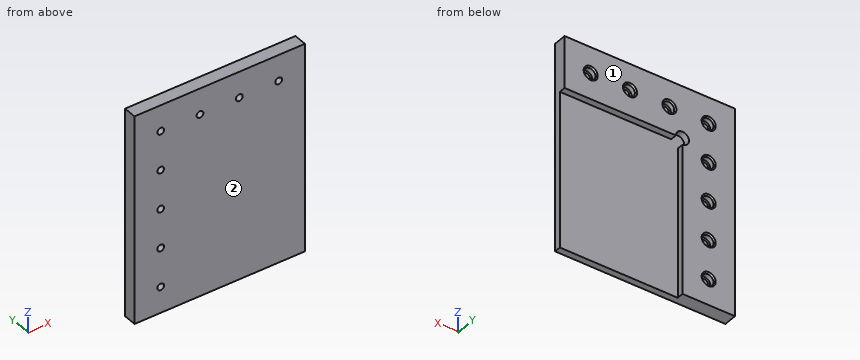
```python
from build123d import *

# Parameters (mm, degrees)
BASE_PLATE_W                    = 82.55
BASE_PLATE_H                    = 101.6
MAIN_BODY_DEPTH                 = 6.35
MOUNTING_HOLES_CBORE_AT_2_COUNT = 2
MOUNTING_HOLES_CBORE_AT_2_PITCH = 19.05
MOUNTING_HOLES_CBORE_AT_3_COUNT = 2
MOUNTING_HOLES_CBORE_AT_3_PITCH = 38.1
MOUNTING_HOLES_CBORE_AT_4_COUNT = 2
MOUNTING_HOLES_CBORE_AT_4_PITCH = 57.15
MOUNTING_HOLES_CBORE_AT_5_COUNT = 2
MOUNTING_HOLES_CBORE_AT_5_PITCH = 19.05
MOUNTING_HOLES_CBORE_AT_6_COUNT = 2
MOUNTING_HOLES_CBORE_AT_6_PITCH = 38.1
MOUNTING_HOLES_CBORE_AT_7_COUNT = 2
MOUNTING_HOLES_CBORE_AT_7_PITCH = 57.15
MOUNTING_HOLES_CBORE_AT_8_COUNT = 2
MOUNTING_HOLES_CBORE_AT_8_PITCH = 76.2
L_AREA_EXCLUSION_W              = 57.15
L_AREA_EXCLUSION_H              = 76.2
L_AREA_STEP_CUT_DEPTH           = 3.175
RELIEF_CIRCLE_SKETCH_R          = 3.175
SUBSTRATE_RELIEF_POCKET_DEPTH   = 3.175


with BuildPart() as part:
    # Base Plate → Main Body (new body)
    with BuildSketch(Plane(origin=(0, 0, 0), x_dir=(1, 0, 0), z_dir=(0, 1, 0))):
        Rectangle(BASE_PLATE_W, BASE_PLATE_H)
    extrude(amount=MAIN_BODY_DEPTH)

    # Hole Profile → Mounting Holes _CBORE (revolve, cut)
    with BuildSketch(Plane(origin=(-28.575, 6.35, 38.1), x_dir=(0, 0, 1), z_dir=(1, 0, 0))):
        Polygon((0, 0), (0, 6.35), (1.63195, 6.35), (1.63195, 2.8448), (2.77876, 2.8448), (2.77876, 0.635), (3.41376, 0), align=None)
    mounting_holes_cbore = revolve(axis=Axis((-28.575, 12.7, 38.1), (0, -1, 0)), mode=Mode.SUBTRACT)

    # Mounting Holes _CBORE at 2: Mounting Holes _CBORE ×2
    with Locations(*[(i * MOUNTING_HOLES_CBORE_AT_2_PITCH, 0, 0) for i in range(1, MOUNTING_HOLES_CBORE_AT_2_COUNT)]):
        add(mounting_holes_cbore, mode=Mode.SUBTRACT)

    # Mounting Holes _CBORE at 3: Mounting Holes _CBORE ×2
    with Locations(*[(i * MOUNTING_HOLES_CBORE_AT_3_PITCH, 0, 0) for i in range(1, MOUNTING_HOLES_CBORE_AT_3_COUNT)]):
        add(mounting_holes_cbore, mode=Mode.SUBTRACT)

    # Mounting Holes _CBORE at 4: Mounting Holes _CBORE ×2
    with Locations(*[(i * MOUNTING_HOLES_CBORE_AT_4_PITCH, 0, 0) for i in range(1, MOUNTING_HOLES_CBORE_AT_4_COUNT)]):
        add(mounting_holes_cbore, mode=Mode.SUBTRACT)

    # Mounting Holes _CBORE at 5: Mounting Holes _CBORE ×2
    with Locations(*[(0, 0, -i * MOUNTING_HOLES_CBORE_AT_5_PITCH) for i in range(1, MOUNTING_HOLES_CBORE_AT_5_COUNT)]):
        add(mounting_holes_cbore, mode=Mode.SUBTRACT)

    # Mounting Holes _CBORE at 6: Mounting Holes _CBORE ×2
    with Locations(*[(0, 0, -i * MOUNTING_HOLES_CBORE_AT_6_PITCH) for i in range(1, MOUNTING_HOLES_CBORE_AT_6_COUNT)]):
        add(mounting_holes_cbore, mode=Mode.SUBTRACT)

    # Mounting Holes _CBORE at 7: Mounting Holes _CBORE ×2
    with Locations(*[(0, 0, -i * MOUNTING_HOLES_CBORE_AT_7_PITCH) for i in range(1, MOUNTING_HOLES_CBORE_AT_7_COUNT)]):
        add(mounting_holes_cbore, mode=Mode.SUBTRACT)

    # Mounting Holes _CBORE at 8: Mounting Holes _CBORE ×2
    with Locations(*[(0, 0, -i * MOUNTING_HOLES_CBORE_AT_8_PITCH) for i in range(1, MOUNTING_HOLES_CBORE_AT_8_COUNT)]):
        add(mounting_holes_cbore, mode=Mode.SUBTRACT)

    # L-Area Exclusion → L-Area Step Cut (cut)
    with BuildSketch(Plane(origin=(0, 6.35, 0), x_dir=(1, 0, 0), z_dir=(0, 1, 0))):
        with Locations((12.7, 12.7)):
            Rectangle(L_AREA_EXCLUSION_W, L_AREA_EXCLUSION_H)
    extrude(amount=-L_AREA_STEP_CUT_DEPTH, mode=Mode.SUBTRACT)

    # Relief Circle Sketch → Substrate Relief Pocket (cut)
    with BuildSketch(Plane(origin=(0, 6.35, 0), x_dir=(1, 0, 0), z_dir=(0, 1, 0))):
        with Locations((-15.875, -25.4)):
            Circle(RELIEF_CIRCLE_SKETCH_R)
    extrude(amount=-SUBSTRATE_RELIEF_POCKET_DEPTH, mode=Mode.SUBTRACT)


solid = part.part
```
Geometry check sheet. Reference: the model listing, model coordinates, mm. Face numbers are marked on the shaded views. Round coordinates to 2 decimals unless told otherwise and drop trailing zeros. Loops run counter-clockwise (first coordinate to the right, second up) from the corner with the lowest first, then second, coordinate; pieces in that order, holes last. Notation, with made-up numbers: (15.5, 15) - (61.5, 15) arc R28 cw to (61.5, 40) - close; hole circle Ø3 at (-7.75, -3.5). An arc over 180 degrees is marked (long way). Write item = value, one per line. Start each with the question number.
1. Section check B-B on y = 4.5. Give the number of separate pieces and of enclosed holes in the cut face, then the cut area to 3 significant figures.
2. Section check D-D on x = -3.5. Enter the section's corners in (y, z) (3 decimals), then the cut area to 3 significant figures.
3. Thickness scan on line 1 (X direction, y = 5.05, z = 38.1) (3 decimals); line 2 (Z direction, x = -28.5, y = 2.25); line 3 (X direction, y = 1.1, z = 38.1) (3 decimals). Record the ranges inside material, lowest first.
4. Mould release check, pull along Y, two halves, no side actions. Record for the marked faces 1 and 2: released by +Y, released by -Y, zero draft, split by the parting line, or undercut.
5. Depth check by flat-ended pin: pin 1 (1.7 mm diameter, centred on x = 29, z = 39, fed in from +Y); pin 2 (2 mm diameter, centred on x = -28.575, z = -38.1, fed in from -Y); pin 3 (6.5 mm diameter, centred on x = -28.575, z = 0, fed in from +Y); pin 4 (1 mm diameter, centred on x = 24.5, y = 4, fed in from -Z). Enter the tip coordinate at first touch or a pass-through.
6. Section check C-C on z = -11.5. Enter the section's corners in (x, y) (3 decimals), then the cut area to 3 significant figures.
7. Section check A-A on z = -38.1. Enter the section's corners in (x, y) (3 decimals).
Working result:
q1.separate_pieces = 1
q1.enclosed_holes = 8
q1.area = 3,810 mm^2
q2.outline = (0, -50.8) - (3.175, -50.8) - (3.175, 25.4) - (6.35, 25.4) - (6.35, 50.8) - (0, 50.8) - close
q2.area = 403 mm^2
q3.line_1 = -41.275 to -31.354, -25.796 to -12.304, -6.746 to 6.746, 12.304 to 25.796, 31.354 to 41.275
q3.line_2 = -50.8 to -39.73, -36.47 to -20.68, -17.42 to -1.63, 1.63 to 17.42, 20.68 to 36.47, 39.73 to 50.8
q3.line_3 = -41.275 to -30.207, -26.943 to -11.157, -7.893 to 7.893, 11.157 to 26.943, 30.207 to 41.275
q4.face_1 = released by +Y
q4.face_2 = released by -Y
q5.pin_1 = 3.51
q5.pin_2 = through
q5.pin_3 = 6.19
q5.pin_4 = 25.4
q6.outline = (-41.275, 0) - (41.275, 0) - (41.275, 3.175) - (-15.875, 3.175) - (-15.875, 6.35) - (-41.275, 6.35) - close
q6.area = 343 mm^2
q7.outline = (-41.275, 0) - (-30.207, 0) - (-30.207, 3.505) - (-31.354, 3.505) - (-31.354, 5.715) - (-31.989, 6.35) - (-41.275, 6.35) - close; (-26.943, 0) - (41.275, 0) - (41.275, 3.175) - (-15.875, 3.175) - (-15.875, 6.35) - (-25.161, 6.35) - (-25.796, 5.715) - (-25.796, 3.505) - (-26.943, 3.505) - close
